Check sheet for the modelled part. Datum: model origin and axes. Units: mm. A direction names the side the tool comes from. Round coordinates to 2 decimals unless told otherwise and drop trailing zeros. Write each loop counter-clockwise with the first axis right and the second up, starting at its lowest first coordinate (ties: lowest second). Pieces come first, ordered by that corner, then holes. Notation, with made-up numbers: (88.25, -39.75) - (122.25, -39.75) arc R30 ccw to (122.25, -14.75) - close; hole circle Ø6 at (66, 48). An arc over 180 degrees is marked (long way). Answer as a JSON object with one key per item and string values. Group by question number.
Item 1: Thickness scan on line 1 (Y direction, x = -17.5, z = 22); line 2 (Y direction, x = -18.5, z = 23); line 3 (X direction, y = -14.5, z = 21.75). Record the ranges inside material, lowest first.
Item 2: Release check for a two-part mould opening along Y. For faces 1 (the cylindrical face through (-4.036, 30.736, 12.353)), 2 (the flat face through (6, 0, 0)), 3 (the cylindrical face through (-20.06, 8.28, 17.79)) record: pulls with the +Y half, pulls with the -Y half, needs draft (parallel to the pull), parting line crosses it, or undercut.
Item 3: Gauge pin test, flat ends, axial feed: P1, Ø8, axis at y = -12, z = 11.5, coming from the -X side; P2, Ø0.9, axis at x = 20.5, y = -9, coming from the +Z side; P3, Ø6, axis at x = 6.5, z = 4.5, coming from the +Y side; P4, Ø1, axis at y = -2, z = 18, coming from the +X side. Record the tip position at first contact, or that the pin passes through.
Item 4: Sectioned sample at C-C on z = 9.75. Record the boundary of the cut face in (x, y), plus the area to 3 significant figures.
Item 5: Sectioned sample at A-A on y = 0. Record the boundary of the cut face in (x, z).
Item 6: Set-up check for faces 4 (the flat face through (4.9, 0, 7)), 5 (the cylindrical face through (-20.155, 10.225, 19.084)), 6 (the flat face through (-15.2, -17, 25)): record each of +Z, -Z, +X, -X, +Y, -Y from which the full face is reachable in a straight line by a thin tool's end or side.
```python
from build123d import *

# Parameters (mm, degrees)
SKETCH_R              = 31
PAD_DEPTH             = 25
SKETCH001_R           = 22.6
POCKET_DEPTH          = 12
SKETCH003_W           = 9.8
SKETCH003_H           = 9.8
POCKET001_DEPTH       = 25.001
SKETCH004_R           = 1.8
PAD001_DEPTH          = 12
POLARPATTERN_COUNT    = 8
SKETCH005_R           = 1.8
PAD002_DEPTH          = 10
POLARPATTERN001_COUNT = 16
CHAMFER_SIZE          = 2
CHAMFER001_SIZE       = 2
CHAMFER002_SIZE       = 0.5
CHAMFER003_SIZE       = 0.29


with BuildPart() as part:
    # Sketch → Pad (new body)
    with BuildSketch(Plane.XY):
        Circle(SKETCH_R)
    extrude(amount=PAD_DEPTH)

    # Sketch001 → Pocket (cut)
    with BuildSketch(Plane.XY.offset(25)):
        Circle(SKETCH001_R)
    extrude(amount=-POCKET_DEPTH, mode=Mode.SUBTRACT)

    # Sketch003 → Pocket001 (cut, through all)
    with BuildSketch(Plane(origin=(0, 0, 0), x_dir=(1, 0, 0), z_dir=(0, 0, -1))):
        Rectangle(SKETCH003_W, SKETCH003_H)
    extrude(amount=-POCKET001_DEPTH, mode=Mode.SUBTRACT)

    # Sketch004 → Pad001 (new body)
    with BuildSketch(Plane.XY.offset(13)):
        with Locations((0, 23.5)):
            Circle(SKETCH004_R)
    pad001 = extrude(amount=PAD001_DEPTH)

    # PolarPattern: Pad001 ×8 about axis
    polarpattern_axis = Axis((0, 0, 13), (0, 0, 1))
    for i in range(1, POLARPATTERN_COUNT):
        add(pad001.rotate(polarpattern_axis, i * 360 / POLARPATTERN_COUNT))

    # Sketch005 → Pad002 (new body)
    with BuildSketch(Plane.XY.offset(13)):
        with Locations((0, 23.5)):
            Circle(SKETCH005_R)
    pad002 = extrude(amount=PAD002_DEPTH)

    # PolarPattern001: Pad002 ×16 about axis
    polarpattern001_axis = Axis((0, 0, 13), (0, 0, 1))
    for i in range(1, POLARPATTERN001_COUNT):
        add(pad002.rotate(polarpattern001_axis, i * 360 / POLARPATTERN001_COUNT))

    # Chamfer
    chamfer_edges = [part.edges().sort_by_distance(p)[0] for p in [
        (-31, 0, 25),
    ]]
    chamfer(chamfer_edges, length=CHAMFER_SIZE)

    # Chamfer001
    chamfer001_edges = [part.edges().sort_by_distance(p)[0] for p in [
        (-31, 0, 0),
    ]]
    chamfer(chamfer001_edges, length=CHAMFER001_SIZE)

    # Chamfer002
    chamfer002_edges = [part.edges().sort_by_distance(p)[0] for p in [
        (-4.9, 0, 0),
        (0, 4.9, 0),
        (4.9, 0, 0),
        (0, -4.9, 0),
    ]]
    chamfer(chamfer002_edges, length=CHAMFER002_SIZE)

    # Chamfer003
    chamfer003_edges = [part.edges().sort_by_distance(p)[0] for p in [
        (8.30423, 20.048186, 23),
        (20.048186, 8.30423, 23),
        (20.048186, -8.30423, 23),
        (8.30423, -20.048186, 23),
        (-8.30423, -20.048186, 23),
        (-20.048186, -8.30423, 23),
        (-20.048186, 8.30423, 23),
        (-8.30423, 20.048186, 23),
    ]]
    chamfer(chamfer003_edges, length=CHAMFER003_SIZE)


solid = part.part
```
Completed:
{
 "1": {"line 1": "-25.59 to -14.3, 14.3 to 25.59", "line 2": "-24.87 to -12.98, 12.98 to 24.87", "line 3": "-27.4 to -17.34, 17.34 to 27.4"},
 "2": {"face 1": "parting line crosses it", "face 2": "needs draft", "face 3": "undercut"},
 "3": {"P1": "x = -29.95", "P2": "z = 25", "P3": "y = 30.8", "P4": "x = 30.96"},
 "4": {"outline": "circle Ø62 at (0, 0); hole (-4.9, -4.9) - (4.9, -4.9) - (4.9, 4.9) - (-4.9, 4.9) - close", "area": "2,920 mm²"},
 "5": {"outline": "(-31, 2) - (-29, 0) - (-5.4, 0) - (-4.9, 0.5) - (-4.9, 13) - (-21.7, 13) - (-21.7, 25) - (-29, 25) - (-31, 23) - close; (4.9, 0.5) - (5.4, 0) - (29, 0) - (31, 2) - (31, 23) - (29, 25) - (21.7, 25) - (21.7, 13) - (4.9, 13) - close"},
 "6": {"face 4": "+Z, -Z", "face 5": "+Z", "face 6": "+Z, +X, -X, +Y, -Y"}
}
